```python
from build123d import *

# Parameters (mm, degrees)
PAD_DEPTH    = 25
SKETCH003_R  = 1.25
POCKET_DEPTH = 10
SKETCH004_R  = 3.35
PAD001_DEPTH = 1


with BuildPart() as pad:
    # Sketch002 → Pad (new body, symmetric)
    with BuildSketch(Plane.XY):
        Polygon((25, 13), (-11.6141486117, -9), (25, -9), align=None)
    extrude(amount=PAD_DEPTH, both=True)


with BuildPart() as pad001:
    # Sketch001 → Revolution001 (revolve)
    with BuildSketch(Plane.XY):
        Polygon((0, -9), (0, -5), (2.05, -5), (2.05, 15), (22, 15), (22, -9), align=None)
    revolve(axis=Axis((0, 0, 0), (0, 1, 0)))

    # Cut: cut Pad
    add(pad.part, mode=Mode.SUBTRACT)

    # Sketch003 → Pocket (cut)
    with BuildSketch(Plane(origin=(0.8924461116, -1.4852797526, 0), x_dir=(0.8571673007, 0.5150380749, 0), z_dir=(0.5150380749, -0.8571673007, 0))):
        with Locations((-4.5, 18)):
            Circle(SKETCH003_R)
        with Locations((2, 18)):
            Circle(SKETCH003_R)
        with Locations((12, -1.5)):
            Circle(SKETCH003_R)
        with Locations((-9, -1.5)):
            Circle(SKETCH003_R)
    extrude(amount=-POCKET_DEPTH, mode=Mode.SUBTRACT)

    # Sketch004 → Pad001 (new body)
    with BuildSketch(Plane(origin=(0.8924461116, -1.4852797526, 0), x_dir=(0.8571673007, 0.5150380749, 0), z_dir=(0.5150380749, -0.8571673007, 0))):
        with Locations((-1.25, 10.5)):
            Circle(SKETCH004_R)
    extrude(amount=PAD001_DEPTH)


solid = pad001.part
```
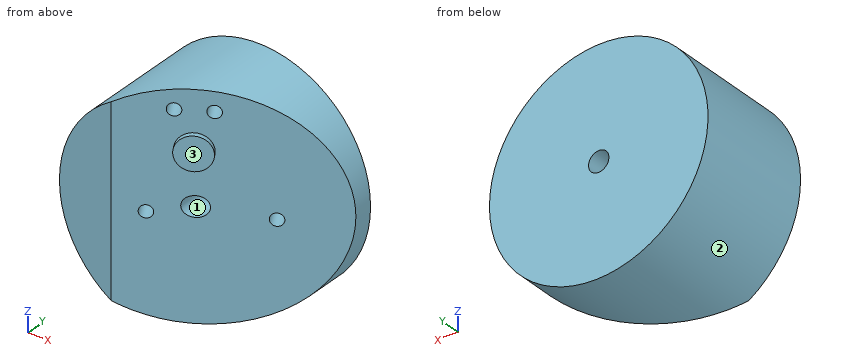
Geometry: final body of the model. Coordinates: model frame, mm. Face numbers are marked on the shaded views. Round coordinates to 2 decimals unless told otherwise and drop trailing zeros. Order: outer loops, then holes, each group sorted by start corner. A loop starts at its lowest first (then second) coordinate and runs counter-clockwise, first axis right, second up. Notation, with made-up numbers: (8, 10.5) -> (54, 10.5) arc R20 ccw to (54, 30.5) -> close; hole circle Ø1 at (35.5, -18). An arc over 180 degrees is marked (long way). Use one line per item in the form item = value.
(1) Section B-B on x = -0.5. Count the separate pieces of the cut face and the enclosed holes in it, and give its area (3 significant figures).
Results list:
separate_pieces = 2
enclosed_holes = 1
area = 691 mm^2
(2) Ray query, probe 1 along X at (y, z) = (1.75, 0); probe 2 along Z at (x, y) = (-10, 0); probe 3 along X at (y, z) = (9, 0). Return the intervals inside material, ascending. Write a range as [from, to].
Results list:
probe_1 = [-22, -2.05], [2.05, 6.28]
probe_2 = [-19.6, -2.67], [-0.33, 19.6]
probe_3 = [-22, -2.05], [2.05, 18.34]
(3) First-contact query: pin 1 Ø1.5 at (x, y) = (-8, 4.5) entering from -Z; pin 2 Ø1 at (y, z) = (-0.5, -11) entering from +X; pin 3 Ø4 at (x, y) = (-7.5, 4.5) entering from -Z. Flat tips, straight axial feed; report the tip coordinate or a pass-through.
Results list:
pin_1 = -20.77
pin_2 = 3.36
pin_3 = -21.3
(4) Draft query along X for the marked faces 1, 2 and 3. Return one class per face: pulls with the +X half, pulls with the -X half, needs draft (parallel to the pull), parting line crosses it, or undercut.
Results list:
face_1 = undercut
face_2 = parting line crosses it
face_3 = pulls with the +X half
(5) Section A-A on z = -4. Return loops of the section in (x, y).
Results list:
outline = (-21.63, -9) -> (-11.61, -9) -> (21.63, 10.98) -> (21.63, 15) -> (-21.63, 15) -> close
(6) Section D-D on z = 16. Return loops of the section in (x, y).
Results list:
outline = (-15.1, -9) -> (-11.61, -9) -> (15.1, 7.05) -> (15.1, 15) -> (-15.1, 15) -> close
